from build123d import *

# Parameters (mm, degrees)
SKETCH1_R           = 42.5
SKETCH1_R_2         = 30.5
SKETCH1_R_3         = 1.5
BOSS_EXTRUDE1_DEPTH = 2
SKETCH2_R           = 1.5
CUT_EXTRUDE1_DEPTH  = 61.137342808
CUT_EXTRUDE2_DEPTH  = 61.137342808
CUT_EXTRUDE3_DEPTH  = 61.137342808
FILLET1_R           = 1


with BuildPart() as part:
    # Sketch1 → Boss-Extrude1 (new body)
    with BuildSketch(Plane(origin=(0, 0, 0), x_dir=(1, 0, 0), z_dir=(0, 1, 0))):
        with Locations(Location((0, 0, 0), (0, 0, 270))):
            Circle(SKETCH1_R)
        with Locations(Location((0, 0, 0), (0, 0, 270))):
            Circle(SKETCH1_R_2, mode=Mode.SUBTRACT)
        with Locations(Location((0, 34.1739971, 0), (0, 0, 270))):
            Circle(SKETCH1_R_3, mode=Mode.SUBTRACT)
        with Locations(Location((-29.672696408, -17.456745562, 0), (0, 0, 270))):
            Circle(SKETCH1_R_3, mode=Mode.SUBTRACT)
        with Locations(Location((29.672696408, -16.717251537, 0), (0, 0, 270))):
            Circle(SKETCH1_R_3, mode=Mode.SUBTRACT)
        with Locations(Location((-32.475952642, 18.75, 0), (0, 0, 270))):
            Circle(SKETCH1_R_3, mode=Mode.SUBTRACT)
        with Locations(Location((0, -37.5, 0), (0, 0, 270))):
            Circle(SKETCH1_R_3, mode=Mode.SUBTRACT)
        with Locations(Location((32.475952642, 18.75, 0), (0, 0, 270))):
            Circle(SKETCH1_R_3, mode=Mode.SUBTRACT)
    extrude(amount=BOSS_EXTRUDE1_DEPTH)

    # Sketch2 → Cut-Extrude1 (cut, through all)
    # profile 1 of 3: a face of its own
    with BuildSketch(Plane(origin=(0, 2, 0), x_dir=(1, 0, 0), z_dir=(0, 1, 0))):
        with BuildLine():
            ThreePointArc((2.523370479, 36.085879061), (0, 36.1739971), (-2.523370479, 36.085879061))
            ThreePointArc((-2.523370479, 36.085879061), (-4.378985632, 33.951238013), (-2.244344584, 32.09562286))
            ThreePointArc((-2.244344584, 32.09562286), (0, 32.1739971), (2.244344584, 32.09562286))
            ThreePointArc((2.244344584, 32.09562286), (4.378985632, 33.951238013), (2.523370479, 36.085879061))
        make_face()
        with Locations((0, 34.1739971)):
            Circle(SKETCH2_R, mode=Mode.SUBTRACT)
    # profile 2 of 3: a face of its own
    with BuildSketch(Plane(origin=(0, 2, 0), x_dir=(1, 0, 0), z_dir=(0, 1, 0))):
        with BuildLine():
            ThreePointArc((-32.608491766, -16.235777693), (-31.396508518, -18.470881554), (-30.031564637, -20.615997137))
            ThreePointArc((-30.031564637, -20.615997137), (-27.250781536, -21.132954915), (-26.733823758, -18.352171814))
            ThreePointArc((-26.733823758, -18.352171814), (-27.948884299, -16.442609571), (-29.027780684, -14.452940586))
            ThreePointArc((-29.027780684, -14.452940586), (-31.709554778, -13.554003599), (-32.608491766, -16.235777693))
        make_face()
        with Locations((-29.672696408, -17.456745562)):
            Circle(SKETCH2_R, mode=Mode.SUBTRACT)
    # profile 3 of 3: a face of its own
    with BuildSketch(Plane(origin=(0, 2, 0), x_dir=(1, 0, 0), z_dir=(0, 1, 0))):
        with BuildLine():
            ThreePointArc((30.104043518, -19.847248501), (31.41518565, -17.69894968), (32.573276155, -15.464423355))
            ThreePointArc((32.573276155, -15.464423355), (31.6243086, -12.799942059), (28.959827303, -13.748909615))
            ThreePointArc((28.959827303, -13.748909615), (27.930207167, -15.735553395), (26.764513869, -17.64553514))
            ThreePointArc((26.764513869, -17.64553514), (27.333422013, -20.416156645), (30.104043518, -19.847248501))
        make_face()
        with Locations((29.672696408, -16.717251537)):
            Circle(SKETCH2_R, mode=Mode.SUBTRACT)
    extrude(amount=-CUT_EXTRUDE1_DEPTH, mode=Mode.SUBTRACT)

    # Sketch3 → Cut-Extrude2 (cut, through all)
    with BuildSketch(Plane(origin=(0, 2, 0), x_dir=(1, 0, 0), z_dir=(0, 1, 0))):
        with BuildLine():
            Line((-29.777028217, 6.601408225), (-33.194064242, 7.358946874))
            ThreePointArc((-33.194064242, 7.358946874), (-29.444863729, 17), (-22.970067059, 25.067429452))
            Line((-22.970067059, 25.067429452), (-20.492564537, 22.58992693))
            ThreePointArc((-20.492564537, 22.58992693), (-26.37548429, 15.316129684), (-29.777028217, 6.601408225))
        make_face()
        with BuildLine():
            Line((20.605501332, 22.486958773), (22.970067059, 25.067429452))
            ThreePointArc((22.970067059, 25.067429452), (29.444863729, 17), (33.194064242, 7.358946874))
            Line((33.194064242, 7.358946874), (29.777028217, 6.601408225))
            ThreePointArc((29.777028217, 6.601408225), (26.413774815, 15.25), (20.605501332, 22.486958773))
        make_face()
        with BuildLine():
            Line((-9.171526885, -29.088366998), (-10.223997183, -32.426376325))
            ThreePointArc((-10.223997183, -32.426376325), (0, -34), (10.223997183, -32.426376325))
            Line((10.223997183, -32.426376325), (9.171526885, -29.088366998))
            ThreePointArc((9.171526885, -29.088366998), (0, -30.5), (-9.171526885, -29.088366998))
        make_face()
    extrude(amount=-CUT_EXTRUDE2_DEPTH, mode=Mode.SUBTRACT)

    # Sketch4 → Cut-Extrude3 (cut, through all)
    with BuildSketch(Plane(origin=(0, 2, 0), x_dir=(1, 0, 0), z_dir=(0, 1, 0))):
        with BuildLine():
            Line((-30.200854727, 4.261264341), (-38.617486372, 5.448829814))
            ThreePointArc((-38.617486372, 5.448829814), (-38.998694951, -0.319048797), (-38.523169542, -6.079918457))
            Line((-38.523169542, -6.079918457), (-30.127094129, -4.754808024))
            ThreePointArc((-30.127094129, -4.754808024), (-30.498979385, -0.249512521), (-30.200854727, 4.261264341))
        make_face()
    extrude(amount=-CUT_EXTRUDE3_DEPTH, mode=Mode.SUBTRACT)

    # Fillet1
    fillet1_edges = [part.edges().sort_by_distance(p)[0] for p in [
        (-20.492564537, 1, -22.58992693),
        (-29.777028217, 1, -6.601408225),
        (-33.194064242, 1, -7.358946874),
        (-22.970067059, 1, -25.067429452),
        (-9.171526885, 1, 29.088366998),
        (9.171526885, 1, 29.088366998),
        (10.223997183, 1, 32.426376325),
        (-10.223997183, 1, 32.426376325),
        (22.970067059, 1, -25.067429452),
        (33.194064242, 1, -7.358946874),
        (29.777028217, 1, -6.601408225),
        (20.605501332, 1, -22.486958773),
        (-30.200854727, 1, -4.261264341),
        (-30.127094129, 1, 4.754808024),
        (-38.523169542, 1, 6.079918457),
        (-38.617486372, 1, -5.448829814),
    ]]
    fillet(fillet1_edges, radius=FILLET1_R)


solid = part.part
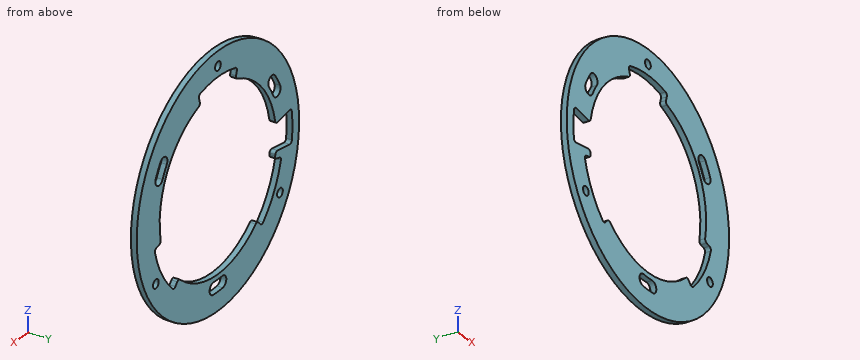
Part model, mm, in its own coordinate system. Round coordinates to 2 decimals unless told otherwise and drop trailing zeros. Loops run counter-clockwise (first coordinate to the right, second up) from the corner with the lowest first, then second, coordinate; pieces in that order, holes last. Notation, with made-up numbers: (-14.75, -1) - (11.25, -1) arc R28 ccw to (11.25, 34) - close; hole circle Ø11 at (60, 79.5). An arc over 180 degrees is marked (long way). Answer as a JSON object with one key per item and string values.
Item 1: Wall check: L1, parallel to Z at x = -28, y = 0.55; L2, parallel to Z at x = -27, y = 0.7; L3, parallel to X at y = 1.2, z = -18.75. Give the ranges that are in metal, low to high.
Output:
{"L1": "-31.97 to -19.29, 12.09 to 16.36, 21.45 to 31.97", "L2": "-32.82 to -20.66, 14.19 to 17.96, 20.93 to 32.82", "L3": "-38.14 to -33.98, -30.98 to -28.36, 28.36 to 30.98, 33.98 to 38.14"}
Item 2: Band-saw the part on A-A on z = 0. List the corners of the cut face in (x, y).
Output:
{"outline": "(-42.5, 0) - (-39, 0) - (-39, 2) - (-42.5, 2) - close; (30.5, 0) - (42.5, 0) - (42.5, 2) - (30.5, 2) - close"}
Item 3: Band-saw the part on D-D on z = 37.5. List the corners of the cut face in (x, y).
Output:
{"outline": "(-20, 0) - (-1.5, 0) - (-1.5, 2) - (-20, 2) - close; (1.5, 0) - (20, 0) - (20, 2) - (1.5, 2) - close"}
Item 4: Band-saw the part on C-C on z = -18.75. List the corners of the cut face in (x, y), plus the area to 3 significant figures.
Output:
{"outline": "(-38.14, 0) - (-33.98, 0) - (-33.98, 2) - (-38.14, 2) - close; (-30.98, 0) - (-28.36, 0) - (-28.36, 2) - (-30.98, 2) - close; (28.36, 0) - (30.98, 0) - (30.98, 2) - (28.36, 2) - close; (33.98, 0) - (38.14, 0) - (38.14, 2) - (33.98, 2) - close", "area": "27.1 mm2"}
Item 5: Pin check, flat tips, straight feed: pin 1 (1 mm diameter, centred on x = 22, y = 1.5, fed in from -Z); pin 2 (6 mm diameter, centred on x = 27.5, z = 9, fed in from -Y). Stop position of each tip, or through.
Output:
{"pin 1": "z = -36.66", "pin 2": "y = 0"}
Item 6: Band-saw the part on B-B on x = 0. List the corners of the cut face in (y, z).
Output:
{"outline": "(0, -42.5) - (2, -42.5) - (2, -36.17) - (0, -36.17) - close; (0, -32.17) - (2, -32.17) - (2, -30.5) - (0, -30.5) - close; (0, 34) - (2, 34) - (2, 36) - (0, 36) - close; (0, 39) - (2, 39) - (2, 42.5) - (0, 42.5) - close"}
